Could you check a few things on this model? Use its own coordinates, in mm. Give positions to 0.01 mm unless a question says otherwise; leave off trailing zeros. Answer as CSV lines item,"result". Start each with the question number.
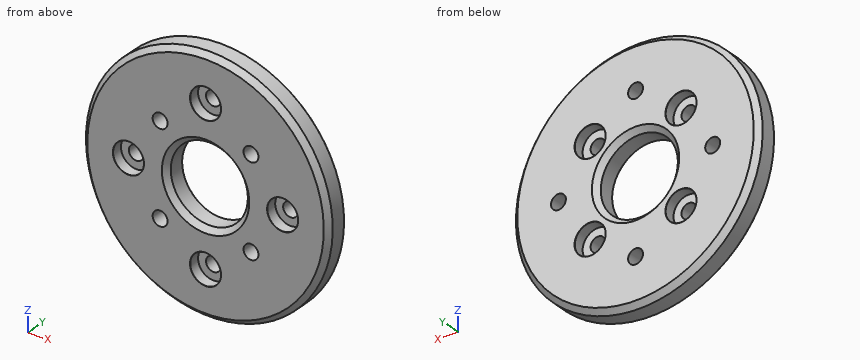
from build123d import *

# Parameters (mm, degrees)
SKETCH1_R               = 24
BOSS_EXTRUDE1_DEPTH     = 5
CUT_EXTRUDE1_DEPTH      = 35.307433597
CUT_EXTRUDE1_DEPTH_BACK = 35.307433597
SKETCH8_R               = 7.5
CHAMFER1_SIZE           = 1
CHAMFER2_SIZE           = 1


# Read off the part's stored shape, not the designer's step: CBORE for M2.5 Pan Head Screw1, CBORE for M2.5 Pan Head Screw2
with BuildPart() as part:
    # Sketch1 → Boss-Extrude1 (new body)
    with BuildSketch(Plane(origin=(0, 0, 0), x_dir=(1, 0, 0), z_dir=(0, 1, 0))):
        with Locations(Location((0, 0, 0), (0, 0, 270))):
            Circle(SKETCH1_R)
    extrude(amount=BOSS_EXTRUDE1_DEPTH)

    # CBORE for M2.5 Pan Head Screw1 outline → CBORE for M2.5 Pan Head Screw1 (revolve, cut)
    with BuildSketch(Plane(origin=(8.838834765, 0, 8.838834765), x_dir=(1, 0, 0), z_dir=(0, 0, 1))):
        Polygon((0, 0), (1.45, 0), (1.45, 2.9), (3, 2.9), (3, 4.975), (3.025, 5), (0, 5), align=None)
    revolve(axis=Axis((8.838834765, 0, 8.838834765), (0, 1, 0)), mode=Mode.SUBTRACT)

    # CBORE for M2.5 Pan Head Screw1 2 outline → CBORE for M2.5 Pan Head Screw1 2 (revolve, cut)
    with BuildSketch(Plane(origin=(-8.838834765, 0, -8.838834765), x_dir=(1, 0, 0), z_dir=(0, 0, 1))):
        Polygon((0, 5), (0, 0), (1.45, 0), (1.45, 2.9), (3, 2.9), (3, 4.975), (3.025, 5), align=None)
    revolve(axis=Axis((-8.838834765, 0, -8.838834765), (0, 1, 0)), mode=Mode.SUBTRACT)

    # CBORE for M2.5 Pan Head Screw1 3 outline → CBORE for M2.5 Pan Head Screw1 3 (revolve, cut)
    with BuildSketch(Plane(origin=(-8.838834765, 0, 8.838834765), x_dir=(1, 0, 0), z_dir=(0, 0, 1))):
        Polygon((0, 5), (0, 0), (1.45, 0), (1.45, 2.9), (3, 2.9), (3, 4.975), (3.025, 5), align=None)
    revolve(axis=Axis((-8.838834765, 0, 8.838834765), (0, 1, 0)), mode=Mode.SUBTRACT)

    # CBORE for M2.5 Pan Head Screw1 4 outline → CBORE for M2.5 Pan Head Screw1 4 (revolve, cut)
    with BuildSketch(Plane(origin=(8.838834765, 0, -8.838834765), x_dir=(1, 0, 0), z_dir=(0, 0, 1))):
        Polygon((0, 5), (0, 0), (1.45, 0), (1.45, 2.9), (3, 2.9), (3, 4.975), (3.025, 5), align=None)
    revolve(axis=Axis((8.838834765, 0, -8.838834765), (0, 1, 0)), mode=Mode.SUBTRACT)

    # CBORE for M2.5 Pan Head Screw2 outline → CBORE for M2.5 Pan Head Screw2 (revolve, cut)
    with BuildSketch(Plane.XY.offset(-15)):
        Polygon((1.45, 2.1), (1.45, 5), (0, 5), (0, 0), (3.025, 0), (3, 0.025), (3, 2.1), align=None)
    revolve(axis=Axis((0, 0, -15), (0, 1, 0)), mode=Mode.SUBTRACT)

    # CBORE for M2.5 Pan Head Screw2 2 outline → CBORE for M2.5 Pan Head Screw2 2 (revolve, cut)
    with BuildSketch(Plane.XY.offset(15)):
        Polygon((0, 0), (3.025, 0), (3, 0.025), (3, 2.1), (1.45, 2.1), (1.45, 5), (0, 5), align=None)
    revolve(axis=Axis((0, 0, 15), (0, 1, 0)), mode=Mode.SUBTRACT)

    # CBORE for M2.5 Pan Head Screw2 3 outline → CBORE for M2.5 Pan Head Screw2 3 (revolve, cut)
    with BuildSketch(Plane(origin=(-15, 0, 0), x_dir=(1, 0, 0), z_dir=(0, 0, 1))):
        Polygon((0, 0), (3.025, 0), (3, 0.025), (3, 2.1), (1.45, 2.1), (1.45, 5), (0, 5), align=None)
    revolve(axis=Axis((-15, 0, 0), (0, 1, 0)), mode=Mode.SUBTRACT)

    # CBORE for M2.5 Pan Head Screw2 4 outline → CBORE for M2.5 Pan Head Screw2 4 (revolve, cut)
    with BuildSketch(Plane(origin=(15, 0, 0), x_dir=(1, 0, 0), z_dir=(0, 0, 1))):
        Polygon((0, 0), (3.025, 0), (3, 0.025), (3, 2.1), (1.45, 2.1), (1.45, 5), (0, 5), align=None)
    revolve(axis=Axis((15, 0, 0), (0, 1, 0)), mode=Mode.SUBTRACT)

    # Sketch8 → Cut-Extrude1 (cut, two sides: drawn at the far end of the back side and taken through both)
    with BuildSketch(Plane(origin=(0, 5, 0), x_dir=(1, 0, 0), z_dir=(0, 1, 0)).offset(-CUT_EXTRUDE1_DEPTH_BACK)):
        with Locations(Location((0, 0, 0), (0, 0, 270))):
            Circle(SKETCH8_R)
    extrude(amount=CUT_EXTRUDE1_DEPTH + CUT_EXTRUDE1_DEPTH_BACK, mode=Mode.SUBTRACT)

    # Chamfer1
    chamfer1_edges = [part.edges().sort_by_distance(p)[0] for p in [
        (0, 5, -7.5),
        (0, 0, -7.5),
    ]]
    chamfer(chamfer1_edges, length=CHAMFER1_SIZE)

    # Chamfer2
    chamfer2_edges = [part.edges().sort_by_distance(p)[0] for p in [
        (0, 0, -24),
        (0, 5, -24),
    ]]
    chamfer(chamfer2_edges, length=CHAMFER2_SIZE)


solid = part.part
1. Imagine slicing it at A-A, the plane z = 0. State how many separate pieces and enclosed holes the cut face has, plus the area to 3 significant figures.
2. Will these pins go through, and if not, where does the flat tip stop? P1, Ø5, axis at x = 8.84, z = 8.84, coming from the +Y side; P2, Ø1.7, axis at x = 0, z = -15, coming from the +Y side; P3, Ø3, axis at x = 16.5, y = 1.5, coming from the -Z side (3 decimals); P4, Ø3, axis at x = 5, y = 4.5, coming from the +Z side.
3. Please list where these lines run through material, in increasing order: line 1 (Y direction, x = 1, z = -17); line 2 (X direction, y = 0.6, z = -5); line 3 (X direction, y = 0.55, z = -15).
Solutions:
1,separate pieces,"4"
1,enclosed holes,"0"
1,area,"119 mm²"
2,P1,"y = 2.9"
2,P2,"through"
2,P3,"z = -18.735"
2,P4,"z = 23.73"
3,line 1,"2.1 to 5"
3,line 2,"-23.06 to -6.12, 6.12 to 23.06"
3,line 3,"-18.15 to -3, 3 to 18.15"
